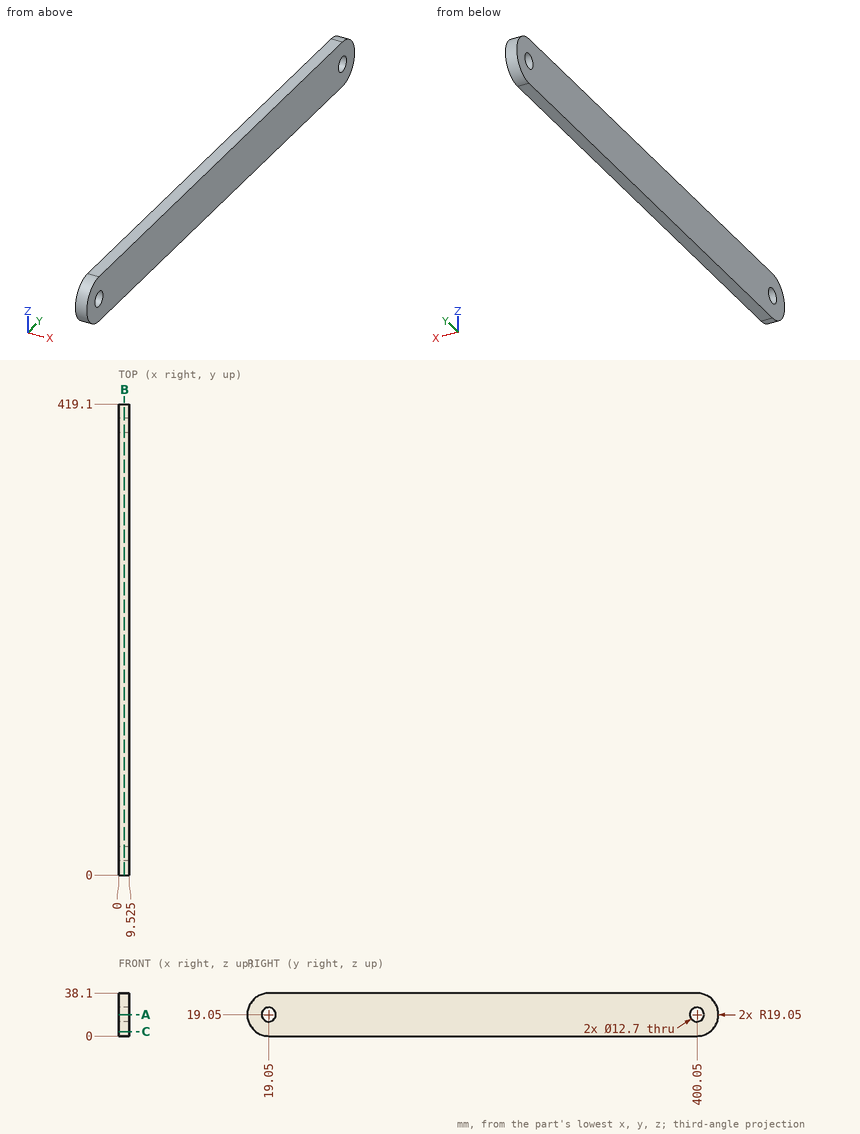
Geometry check sheet. Reference: drawing and pictorial views, mm from the part's lowest x, y, z. Round coordinates to 2 decimals unless told otherwise and drop trailing zeros. Write each loop counter-clockwise with the first axis right and the second up, starting at its lowest first coordinate (ties: lowest second). Pieces come first, ordered by that corner, then holes.
1. Section check A-A on z = 19.05. Enter the section's corners in (x, y) (3 decimals), plus the area to 3 significant figures.
2. Gauge pin test, flat ends, axial feed: P1, Ø5, axis at x = 8.5, z = 11, coming from the -Y side; P2, Ø3, axis at x = 5.5, z = 6.5, coming from the +Y side; P3, Ø1, axis at x = 7, z = 24, coming from the +Y side. Record the tip position at first contact, or that the pin passes through.
3. Section check B-B on x = 5.25. Enter the section's corners in (y, z), plus the area to 3 significant figures.
4. Scan lines: L1, parallel to Z at x = 3.25, y = 400.05; L2, parallel to Y at x = 1.5, z = 18; L3, parallel to Y at x = 8.75, z = 14. Record each from-to range of solid material in increasing order.
5. Section check C-C on z = 4. Enter the section's corners in (x, y) (3 decimals).
Answer:
1. outline: (0, 0) - (9.525, 0) - (9.525, 12.7) - (0, 12.7) - close; (0, 25.4) - (9.525, 25.4) - (9.525, 393.7) - (0, 393.7) - close; (0, 406.4) - (9.525, 406.4) - (9.525, 419.1) - (0, 419.1) - close
1. area: 3,750 mm2
2. P1: stops at y = 0.83
2. P2: stops at y = 415.57
2. P3: stops at y = 418.57
3. outline: (19.05, 0) - (400.05, 0) arc R19.05 ccw to (400.05, 38.1) - (19.05, 38.1) arc R19.05 ccw to start; hole circle Ø12.7 at (19.05, 19.05); hole circle Ø12.7 at (400.05, 19.05)
3. area: 15,400 mm2
4. L1: z = 0 to 12.7, 25.4 to 38.1
4. L2: y = 0.03 to 12.79, 25.31 to 393.79, 406.31 to 419.07
4. L3: y = 0.68 to 15.2, 22.9 to 396.2, 403.9 to 418.42
5. outline: (0, 7.371) - (9.525, 7.371) - (9.525, 411.729) - (0, 411.729) - close
